For this review, use the dimensioned drawing (mm, ordinates from the lowest corner) and the shaded views. Coordinates: 2 decimals unless noted, no trailing zeros. Write each loop counter-clockwise with the first axis right and the second up, starting at its lowest first coordinate (ties: lowest second). Pieces come first, ordered by that corner, then holes. Notation, with made-up numbers: (-5, 47) - (38, 47) arc R11 ccw to (38, 60) - close; hole circle Ø10 at (-20, 47.25). An arc over 180 degrees is marked (long way). Answer as a JSON object with one key per item and string values.
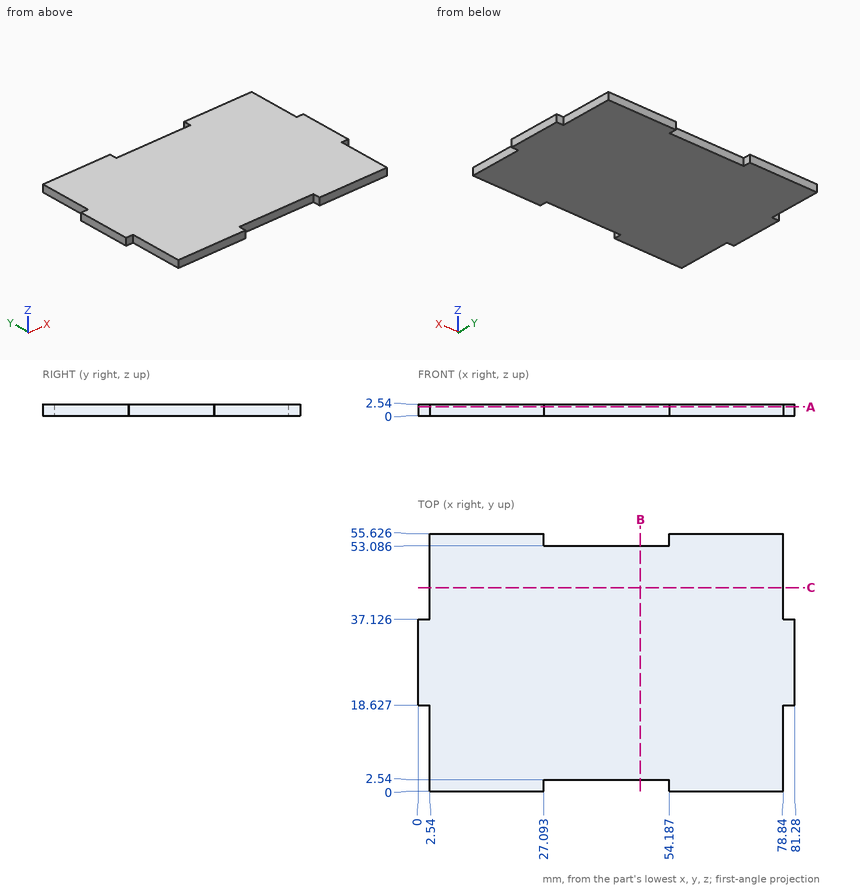
(1) For pin 1 (1.3 mm diameter, centred on y = 7, z = 1, fed in from +X); pin 2 (1.2 mm diameter, centred on x = 80.5, z = 1, fed in from -Y); pin 3 (1.3 mm diameter, centred on y = 54, z = 1.5, fed in from -X), all flat-tipped, find the tip position at first contact; note any pin that passes through.
Solved:
{"pin 1": "stops at x = 78.84", "pin 2": "stops at y = 18.63", "pin 3": "stops at x = 2.54"}
(2) Take a section at C-C, the plane y = 44. Write out the cut boundary in (x, z).
Solved:
{"outline": "(2.54, 0) - (78.84, 0) - (78.84, 2.54) - (2.54, 2.54) - close"}
(3) Take a section at A-A, the plane z = 1.9. Write out the cut boundary in (x, y), and give its area (3 significant figures).
Solved:
{"outline": "(0, 18.63) - (2.54, 18.63) - (2.54, 0) - (27.09, 0) - (27.09, 2.54) - (54.19, 2.54) - (54.19, 0) - (78.84, 0) - (78.84, 18.63) - (81.28, 18.63) - (81.28, 37.13) - (78.84, 37.13) - (78.84, 55.63) - (54.19, 55.63) - (54.19, 53.09) - (27.09, 53.09) - (27.09, 55.63) - (2.54, 55.63) - (2.54, 37.13) - (0, 37.13) - close", "area": "4,200 mm^2"}
(4) To check wall thickness, follow line 1 (Y direction, x = 50.5, z = 1); line 2 (X direction, y = 13.5, z = 0.8). State the ranges of each line that lie inside material, in increasing order. Write a range as from..to.
Solved:
{"line 1": "y = 2.54..53.09", "line 2": "x = 2.54..78.84"}
(5) Take a section at B-B, the plane x = 48. Write out the cut boundary in (y, z), and give its area (3 significant figures).
Solved:
{"outline": "(2.54, 0) - (53.09, 0) - (53.09, 2.54) - (2.54, 2.54) - close", "area": "128 mm^2"}
